```python
from build123d import *

# Parameters (mm, degrees)
CROQUIS1_W              = 7.7
CROQUIS1_H              = 7.7
SALIENTE_EXTRUIR1_DEPTH = 2.5
CROQUIS2_R              = 1.4
SALIENTE_EXTRUIR2_DEPTH = 7.5
SALIENTE_EXTRUIR3_START = 2.5
CROQUIS7_R              = 1.4
SALIENTE_EXTRUIR3_DEPTH = 2.5
CROQUIS6_R              = 0.6
CORTAR_EXTRUIR1_DEPTH   = 14.634331667


with BuildPart() as part:
    # Croquis1 → Saliente-Extruir1 (new body)
    with BuildSketch(Plane.XY):
        Rectangle(CROQUIS1_W, CROQUIS1_H)
    extrude(amount=SALIENTE_EXTRUIR1_DEPTH)

    # Croquis2 → Saliente-Extruir2 (add)
    with BuildSketch(Plane(origin=(0, 0, 0), x_dir=(-1, 0, 0), z_dir=(0, 0, -1))):
        Circle(CROQUIS2_R)
    extrude(amount=SALIENTE_EXTRUIR2_DEPTH)

    # Recubrir2: read off the stored shape, not the designer's step
    # Recubrir2: loft between two sections, ruled curve by curve
    recubrir2_from = [
        Edge.make_bspline([(-0.33839724, 1.767904779, -2.5), (3.197412318, 2.44469926, -2.5), (3.874206798, -1.091110298, -2.5), (0.33839724, -1.767904779, -2.5), (-3.197412318, -2.44469926, -2.5), (-3.874206798, 1.091110298, -2.5), (-0.33839724, 1.767904779, -2.5)], [0, 0, 0, 0, 0.5, 0.5, 0.5, 1, 1, 1, 1], 3, [1, 0.333333333, 0.333333333, 1, 0.333333333, 0.333333333, 1]),
    ]
    recubrir2_to = [
        Edge.make_bspline([(-0.867767345, 1.09862634, -6), (1.329485334, 2.83416103, -6), (3.065020025, 0.636908351, -6), (0.867767345, -1.09862634, -6), (-1.329485334, -2.83416103, -6), (-3.065020025, -0.636908351, -6), (-0.867767345, 1.09862634, -6)], [0, 0, 0, 0, 0.5, 0.5, 0.5, 1, 1, 1, 1], 3, [1, 0.333333333, 0.333333333, 1, 0.333333333, 0.333333333, 1]),
    ]
    recubrir2 = Solid(Shell([*[Face.make_surface_from_curves(recubrir2_from[k], recubrir2_to[k]) for k in range(1)], Face(Wire(recubrir2_from)), Face(Wire(recubrir2_to))]))
    add(recubrir2)

    # Croquis7 → Saliente-Extruir3 (add)
    with BuildSketch(Plane.XY.offset(2.5).offset(SALIENTE_EXTRUIR3_START)):
        with Locations(Location((0, 0, 0), (0, 0, 180))):
            Circle(CROQUIS7_R)
    extrude(amount=-SALIENTE_EXTRUIR3_DEPTH)

    # Croquis6 → Cortar-Extruir1 (cut, through all)
    with BuildSketch(Plane(origin=(0, 0, -7.5), x_dir=(-1, 0, 0), z_dir=(0, 0, -1))):
        Circle(CROQUIS6_R)
    extrude(amount=-CORTAR_EXTRUIR1_DEPTH, mode=Mode.SUBTRACT)


solid = part.part
```
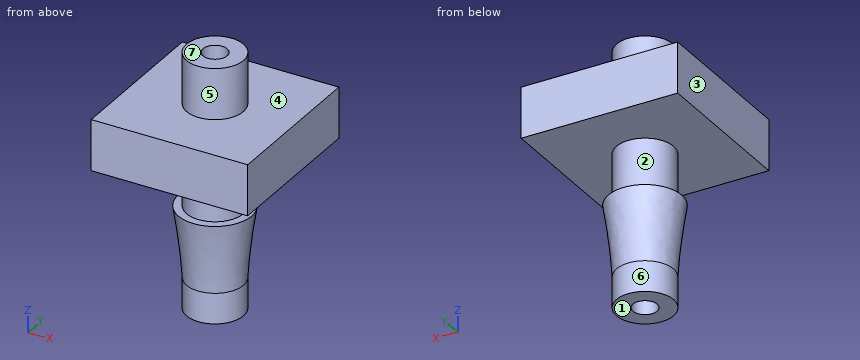
The model under review builds one solid part; all positions refer to its coordinate system, in mm. Face numbers are marked on the shaded views. A direction names the side the tool comes from. Round coordinates to 2 decimals unless told otherwise and drop trailing zeros. Order: outer loops, then holes, each group sorted by start corner. A loop starts at its lowest first (then second) coordinate and runs counter-clockwise, first axis right, second up. Notation, with made-up numbers: (-34.5, -30) -> (18.5, -30) arc R16 cw to (18.5, -7) -> close; hole circle Ø11 at (57.25, 18.5). An arc over 180 degrees is marked (long way). Use a Markdown table: item, result.
Q1. We need section B-B on x = -3.25. Write out the cut boundary in (y, z), then the cut area to 4 significant figures.
Values:
| item | result |
|---|---|
| outline | (-3.85, 0) -> (3.85, 0) -> (3.85, 2.5) -> (-3.85, 2.5) -> close |
| area | 19.25 mm^2 |
Q2. Clearance check with flat-ended pins moving along their axes: P1, Ø1.1, axis at x = 0, y = 0, coming from the -Z side; P2, Ø2, axis at y = -2, z = -4, coming from the -X side. State where each tip first meets the part, or that it passes through.
Values:
| item | result |
|---|---|
| P1 | passes through |
| P2 | stops at x = -1.25 |
Q3. Mouldability with a two-part tool opening along Z and no side actions: class the marked faces 1, 2, 3 and 4 as +Z half, -Z half, draft (parallel to the pull), parting line (faces both ways), or undercut.
Values:
| item | result |
|---|---|
| face 1 | -Z half |
| face 2 | undercut |
| face 3 | draft |
| face 4 | +Z half |
Q4. Tool access review of the marked faces 5, 6 and 7: name each direction out of +Z, -Z, +X, -X, +Y, -Y from which nothing blocks a thin tool from reaching the whole face with its end or side.
Values:
| item | result |
|---|---|
| face 5 | +Z |
| face 6 | -Z |
| face 7 | +Z, +X, -X, +Y, -Y |
Q5. For line 1 (Y direction, x = 0, z = -1.75); line 2 (Y direction, x = 0, z = 1.25); line 3 (Z direction, x = 3, y = -1.5), list the stretches that pass through material, from the lowest coordinate up.
Values:
| item | result |
|---|---|
| line 1 | y = -1.4 to -0.6, 0.6 to 1.4 |
| line 2 | y = -3.85 to -0.6, 0.6 to 3.85 |
| line 3 | z = 0 to 2.5 |
Q6. We need section A-A on z = -1. Write out the cut boundary in (x, y).
Values:
| item | result |
|---|---|
| outline | circle Ø2.8 at (0, 0); hole circle Ø1.2 at (0, 0) |
